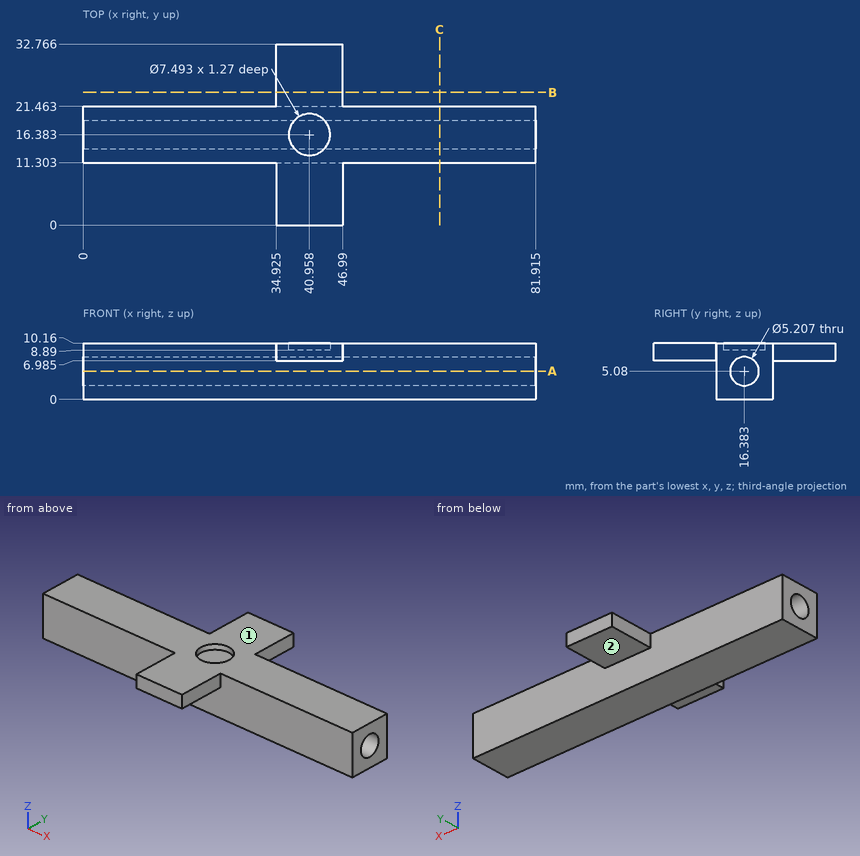
For this review, use the dimensioned drawing (mm, ordinates from the lowest corner) and the shaded views. A direction names the side the tool comes from. Round coordinates to 2 decimals unless told otherwise and drop trailing zeros. Write each loop counter-clockwise with the first axis right and the second up, starting at its lowest first coordinate (ties: lowest second). Pieces come first, ordered by that corner, then holes. Notation, with made-up numbers: M 55.25,54.5 L 65.25,54.5 A21 ccw 65.25,74.5 Z; hole C 33,41 d2. An arc over 180 degrees is marked long. Use CSV: the item, a comma, the result in double quotes. Start each with the question number.
(1) Clearance check with flat-ended pins moving along their axes: P1, Ø6, axis at x = 50, z = 3, coming from the -Y side; P2, Ø4, axis at y = 28.5, z = 7.5, coming from the +X side; P3, Ø3.5, axis at x = 38, y = 29.5, coming from the -Z side (1 decimal). State where each tip first meets the part, or that it passes through.
(2) We need section B-B, the plane y = 24. State the section outline as (x, z) points (1 decimal).
(3) We need section C-C, the plane x = 64.5. State the section outline as (y, z) points.
(4) We need section A-A, the plane z = 5.08. State the section outline as (x, y) points (1 decimal).
(5) For line 1 along Y through (x, z) = (43, 5.08); line 2 along Y through (x, z) = (29, 1.5); line 3 along Z through (x, y) = (42.5, 28.5) (1 decimal), list the stretches that pass through material, from the lowest coordinate up.
(6) Tool access review of the marked faces 1 and 2: name each direction out of +Z, -Z, +X, -X, +Y, -Y from which nothing blocks a thin tool from reaching the whole face with its end or side.
Findings:
1,P1,"y = 11.3"
1,P2,"x = 46.99"
1,P3,"z = 7"
2,outline,"M 34.9,7 L 47,7 L 47,10.2 L 34.9,10.2 Z"
3,outline,"M 11.3,0 L 21.46,0 L 21.46,10.16 L 11.3,10.16 Z; hole C 16.38,5.08 d5.21"
4,outline,"M 0,11.3 L 81.9,11.3 L 81.9,13.8 L 0,13.8 Z; M 0,19 L 81.9,19 L 81.9,21.5 L 0,21.5 Z"
5,line 1,"11.3 to 13.78, 18.99 to 21.46"
5,line 2,"11.3 to 21.46"
5,line 3,"7 to 10.2"
6,face 1,"+Z, +X, -X, +Y, -Y"
6,face 2,"-Z, +X, -X, +Y"
